```python
from build123d import *

# Parameters (mm, degrees)
BOSS_EXTRUDE1_DEPTH = 1.524


with BuildPart() as part:
    # Sketch1 → Boss-Extrude1 (new body)
    with BuildSketch(Plane.XY):
        with BuildLine():
            Line((121.523623664, 0), (120.01155741, 0))
            ThreePointArc((120.01155741, 0), (119.847826563, 0.036974987), (119.71587496, 0.140723308))
            ThreePointArc((119.71587496, 0.140723308), (119.624223582, 0.270551073), (119.550930958, 0.411559635))
            ThreePointArc((119.550930958, 0.411559635), (120.718745933, 1.154856432), (122.0741261, 1.436328542))
            ThreePointArc((122.0741261, 1.436328542), (125.07411423, 0.615177069), (128.177782779, 0.411559635))
            ThreePointArc((128.177782779, 0.411559635), (129.131308323, 0.819549331), (129.965124825, 1.436328542))
            ThreePointArc((129.965124825, 1.436328542), (129.325202776, -0.025891409), (127.908964253, -0.762))
            ThreePointArc((127.908964253, -0.762), (129.325202776, -1.498108591), (129.965124825, -2.960328542))
            ThreePointArc((129.965124825, -2.960328542), (129.131308323, -2.343549331), (128.177782779, -1.935559635))
            ThreePointArc((128.177782779, -1.935559635), (125.07411423, -2.139177069), (122.0741261, -2.960328542))
            ThreePointArc((122.0741261, -2.960328542), (120.718745933, -2.678856432), (119.550930958, -1.935559635))
            ThreePointArc((119.550930958, -1.935559635), (119.624223582, -1.794551073), (119.71587496, -1.664723308))
            ThreePointArc((119.71587496, -1.664723308), (119.847826563, -1.560974987), (120.01155741, -1.524))
            Line((120.01155741, -1.524), (121.523623664, -1.524))
            Line((121.523623664, -1.524), (121.523623664, 0))
        make_face()
    extrude(amount=BOSS_EXTRUDE1_DEPTH)


solid = part.part
```
Check sheet for the modelled part. Datum: model origin and axes. Units: mm. A direction names the side the tool comes from. Coordinates: 2 decimals unless noted, no trailing zeros. Write each loop counter-clockwise with the first axis right and the second up, starting at its lowest first coordinate (ties: lowest second). Pieces come first, ordered by that corner, then holes. Notation, with made-up numbers: (57.25, -33) - (74.25, -33) arc R13 ccw to (74.25, -13) - close; hole circle Ø3 at (46.5, 47). An arc over 180 degrees is marked (long way). One line per question, with ' | ' between items.
Item 1: Sectioned sample at D-D on y = -0.6. Record the boundary of the cut face in (x, z), plus the area to 3 significant figures.
Determined:
outline: (121.52, 0) - (128.5, 0) - (128.5, 1.52) - (121.52, 1.52) - close | area: 10.6 mm2
Item 2: Thickness scan on line 1 (Y direction, x = 120.5, z = 0.55); line 2 (Y direction, x = 129.25, z = 1.2); line 3 (Y direction, x = 123.25, z = 0.9). Record the ranges inside material, lowest first. Write a range as [from, to].
Determined:
line 1: y = [-2.58, -1.52], [0, 1.06] | line 2: y = [-2.41, -1.42], [-0.1, 0.89] | line 3: y = [-2.56, 1.04]
Item 3: Mould release check, pull along Y, two halves, no side actions. Record for faces 1 (the face through (129.34, -0.01, 0.75)), 2 (the face through (125, -1, 0)), 3 (the face through (129.14, -2.35, 0.75)): pulls with the +Y half, pulls with the -Y half, needs draft (parallel to the pull), parting line crosses it, or undercut.
Determined:
face 1: undercut | face 2: needs draft | face 3: pulls with the -Y half
Item 4: Sectioned sample at C-C on x = 121.25. Record the boundary of the cut face in (y, z).
Determined:
outline: (-2.85, 0) - (-1.52, 0) - (-1.52, 1.52) - (-2.85, 1.52) - close; (0, 0) - (1.33, 0) - (1.33, 1.52) - (0, 1.52) - close
Item 5: Gauge pin test, flat end, axial feed: P1, Ø0.5, axis at y = -0.5, z = 1, coming from the -X side. Record the tip position at first contact, or that the pin passes through.
Determined:
P1: stops at x = 121.52
Item 6: Sectioned sample at A-A on z = 0.6. Record the boundary of the cut face in (x, y) (3 decimals), plus the area to 3 significant figures.
Determined:
outline: (119.551, -1.936) arc R3.844 ccw to (122.074, -2.96) arc R15.45 cw to (128.178, -1.936) arc R4.469 cw to (129.965, -2.96) arc R2.397 ccw to (127.909, -0.762) arc R2.397 ccw to (129.965, 1.436) arc R4.469 cw to (128.178, 0.412) arc R15.45 cw to (122.074, 1.436) arc R3.844 ccw to (119.551, 0.412) arc R1.175 ccw to (119.716, 0.141) arc R0.381 ccw to (120.012, 0) - (121.524, 0) - (121.524, -1.524) - (120.012, -1.524) arc R0.381 ccw to (119.716, -1.665) arc R1.175 ccw to start | area: 27.7 mm2
Item 7: Sectioned sample at B-B on y = 0.85. Record the boundary of the cut face in (x, z), plus the area to 3 significant figures.
Determined:
outline: (120.12, 0) - (123.94, 0) - (123.94, 1.52) - (120.12, 1.52) - close; (129.18, 0) - (129.85, 0) - (129.85, 1.52) - (129.18, 1.52) - close | area: 6.83 mm2
Item 8: Access from +Z, -Z, +X, -X, +Y, -Y to the whole of each face (thin tool, end or side, straight path). Record for faces 4 (the face through (129.1, 0.8, 0.8)), 5 (the face through (120.737, -2.686, 0.751)), 6 (the face through (125, -1, 1.524)), 7 (the face through (125.12, -2.13, 0.75)), 8 (the face through (121.524, -1, 1)).
Determined:
face 4: +Z, -Z, +Y | face 5: +Z, -Z, -X, -Y | face 6: +Z, +X, -X, +Y, -Y | face 7: +Z, -Z, -Y | face 8: +Z, -Z, -X
